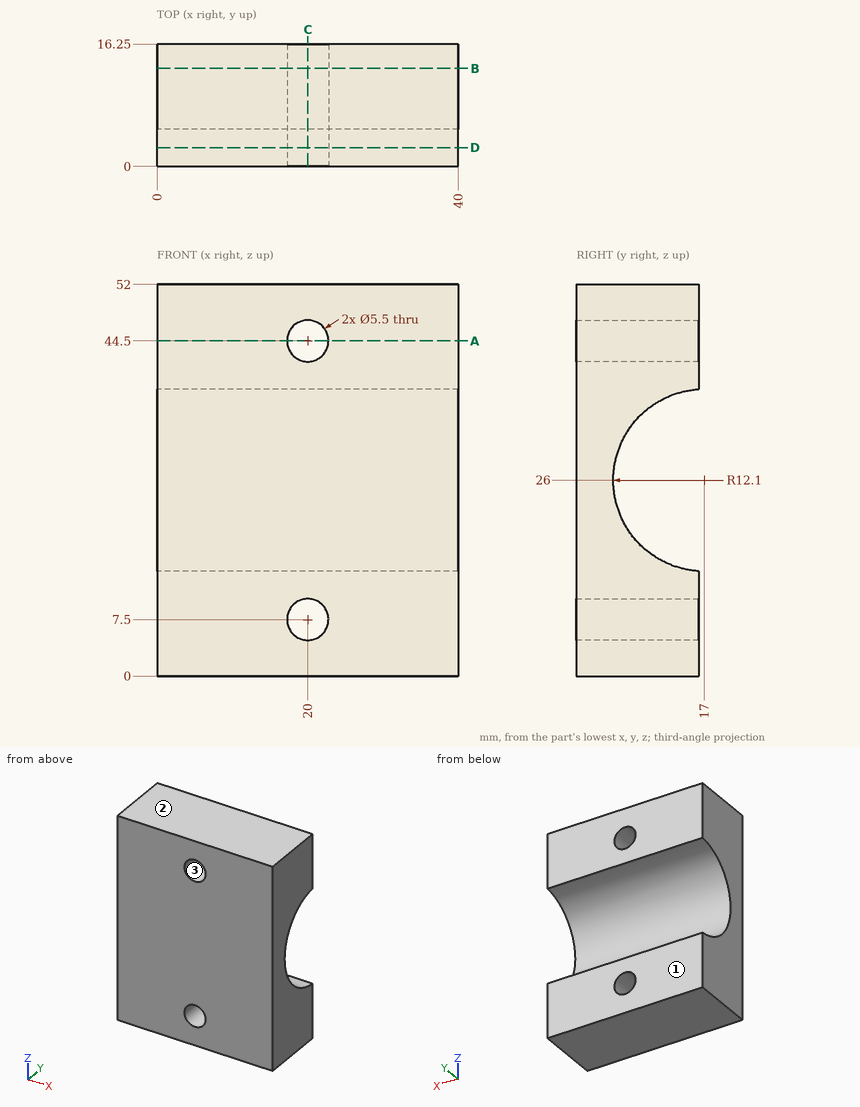
The figure shows three views and two pictorial views of one solid part (mm, origin at its lowest corner). Answer the questions. Coordinates: 2 decimals unless noted, no trailing zeros. Write each loop counter-clockwise with the first axis right and the second up, starting at its lowest first coordinate (ties: lowest second). Pieces come first, ordered by that corner, then holes. Notation, with made-up numbers: (46, 1.25) -> (76, 1.25) arc R14 cw to (76, 6.25) -> close; hole circle Ø3 at (11.5, 73.25). An arc over 180 degrees is marked (long way). Return JSON: item names as keys, results as strings.
1. A cutting plane is placed at D-D (y = 2.5). Determine the outline of the cut face in (x, z).
Found:
{"outline": "(0, 0) -> (40, 0) -> (40, 52) -> (0, 52) -> close; hole circle Ø5.5 at (20, 7.5); hole circle Ø5.5 at (20, 44.5)"}
2. Find the intervals of material crossed by line 1 along Z through (x, y) = (20, 3.5); line 2 along X through (y, z) = (3.75, 7.5); line 3 along Z through (x, y) = (22.5, 15.5), in increasing order. Write a range as from..to.
Found:
{"line 1": "0..4.75, 10.25..41.75, 47.25..52", "line 2": "0..17.25, 22.75..40", "line 3": "0..6.35, 8.65..13.99, 38.01..43.35, 45.65..52"}
3. A cutting plane is placed at C-C (x = 20). Determine the outline of the cut face in (y, z).
Found:
{"outline": "(0, 0) -> (16.25, 0) -> (16.25, 4.75) -> (0, 4.75) -> close; (0, 10.25) -> (16.25, 10.25) -> (16.25, 13.92) arc R12.1 cw to (16.25, 38.08) -> (16.25, 41.75) -> (0, 41.75) -> close; (0, 47.25) -> (16.25, 47.25) -> (16.25, 52) -> (0, 52) -> close"}
4. A cutting plane is placed at B-B (y = 13). Determine the outline of the cut face in (x, z), and give its area (3 significant figures).
Found:
{"outline": "(0, 0) -> (40, 0) -> (40, 14.58) -> (0, 14.58) -> close; (0, 37.42) -> (40, 37.42) -> (40, 52) -> (0, 52) -> close; hole circle Ø5.5 at (20, 7.5); hole circle Ø5.5 at (20, 44.5)", "area": "1,120 mm2"}
5. A cutting plane is placed at A-A (z = 44.5). Determine the outline of the cut face in (x, y).
Found:
{"outline": "(0, 0) -> (17.25, 0) -> (17.25, 16.25) -> (0, 16.25) -> close; (22.75, 0) -> (40, 0) -> (40, 16.25) -> (22.75, 16.25) -> close"}
6. Determine the mould class of the marked faces 1, 2 and 3 for opening direction Z: pulls with the +Z half, pulls with the -Z half, needs draft (parallel to the pull), parting line crosses it, or undercut.
Found:
{"face 1": "needs draft", "face 2": "pulls with the +Z half", "face 3": "undercut"}
7. Each of these flat-tipped pins is pushed along its axis until it touches: P1, Ø4.5, axis at x = 20, z = 7.5, coming from the +Y side; P2, Ø4, axis at x = 32.5, z = 30.5, coming from the +Y side. Where does it stop, or does it pass through?
Found:
{"P1": "through", "P2": "y = 6.79"}
